from build123d import *

# Parameters (mm, degrees)
F3_R     = 33.25
F4_DEPTH = 6
F5_R     = 33.25
F5_R_2   = 27.25
F6_DEPTH = 76
F7_D     = 5
F8_R     = 1


with BuildPart() as f4:
    # F3 (on Top) → F4 (new body)
    with BuildSketch(Plane.XY):
        Circle(F3_R)
    extrude(amount=F4_DEPTH)

    # F5 (on face) → F6 (join)
    with BuildSketch(Plane.XY.offset(6)):
        Circle(F5_R)
        Circle(F5_R_2, mode=Mode.SUBTRACT)
    extrude(amount=F6_DEPTH)

    # F7 (through all)
    with Locations(Plane(origin=(0, 0, 0), x_dir=(1, 0, 0), z_dir=(0, 0, -1))):
        with Locations((-15.125, -15.125), (15.125, -15.125), (15.125, 15.125), (-15.125, 15.125)):
            Hole(F7_D / 2)

    # F8
    f8_edges = [f4.edges().sort_by_distance(p)[0] for p in [
        (-33.25, 0, 0),
        (-33.25, 0, 82),
    ]]
    fillet(f8_edges, radius=F8_R)


solid = f4.part
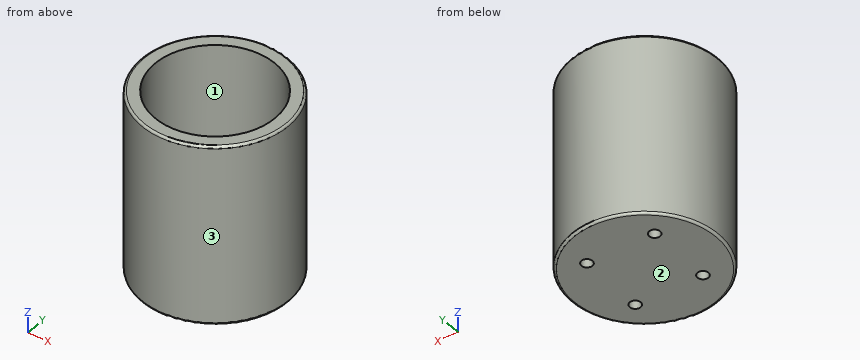
Verification items for the finished model (mm, model axes). Face numbers are marked on the shaded views. Coordinates: 2 decimals unless noted, no trailing zeros. Order: outer loops, then holes, each group sorted by start corner. A loop starts at its lowest first (then second) coordinate and runs counter-clockwise, first axis right, second up. Notation, with made-up numbers: M -30.5,57 L -2.5,57 A21 cw -2.5,63 Z; hole C 83,56 d4. An arc over 180 degrees is marked long. One line per item, written item: value. Start each with the question number.
Item 1: Scan lines: probe 1 along Y at (x, z) = (1, 14); probe 2 along X at (y, z) = (6.5, 49); probe 3 along Z at (x, y) = (-5, -9.5). Record each from-to range of solid material in increasing order.
Item 2: Mould release check, pull along Y, two halves, no side actions. Record for the marked faces 1, 2 and 3: released by +Y, released by -Y, zero draft, split by the parting line, or undercut.
Item 3: Gauge pin test, flat ends, axial feed: pin 1 (4 mm diameter, centred on x = -21.5, z = 63, fed in from +Y); pin 2 (12 mm diameter, centred on x = -3, y = 11, fed in from +Z); pin 3 (1.5 mm diameter, centred on x = -10.5, z = 71, fed in from +Y); pin 4 (2 mm diameter, centred on x = 12, y = -23.5, fed in from +Z). Record the tip position at first contact, or that the pin passes through.
Item 4: Sectioned sample at A-A (x = 0). Enter the section's corners in (y, z), then the cut area to 3 significant figures.
Item 5: Sectioned sample at C-C (z = 18). Enter the section's corners in (x, y).
Conclusion:
1. probe 1: y = -33.23 to -27.23, 27.23 to 33.23
1. probe 2: x = -32.61 to -26.46, 26.46 to 32.61
1. probe 3: z = 0 to 6
2. face 1: undercut
2. face 2: zero draft
2. face 3: split by the parting line
3. pin 1: stops at y = 26.93
3. pin 2: stops at z = 6
3. pin 3: stops at y = 31.79
3. pin 4: stops at z = 82
4. outline: M -33.25,1 A1 ccw -32.25,0 L 32.25,0 A1 ccw 33.25,1 L 33.25,81 A1 ccw 32.25,82 L 27.25,82 L 27.25,6 L -27.25,6 L -27.25,82 L -32.25,82 A1 ccw -33.25,81 Z
4. area: 1,310 mm^2
5. outline: C 0,0 d66.5; hole C 0,0 d54.5
